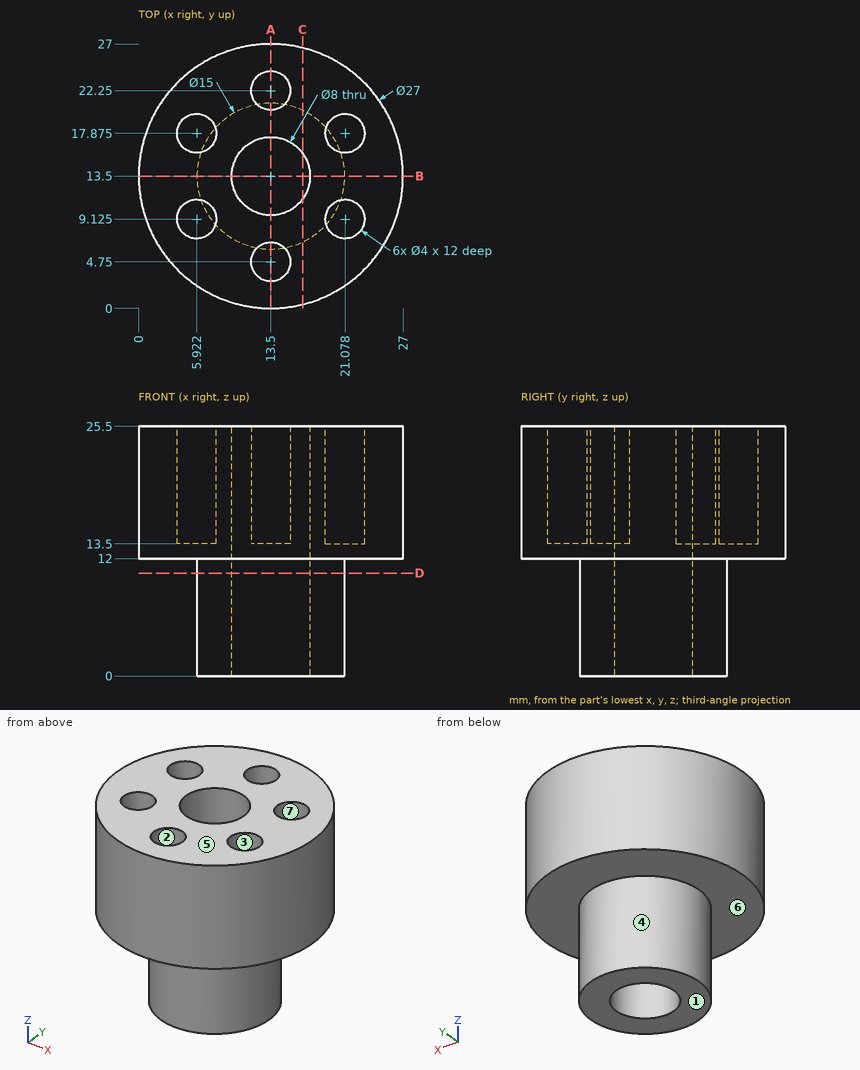
Could you check a few things on this drawing? It's one solid part, dimensions in mm from its lowest x, y, z. A direction names the side the tool comes from. Coordinates: 2 decimals unless noted, no trailing zeros. Order: outer loops, then holes, each group sorted by start corner. A loop starts at its lowest first (then second) coordinate and runs counter-clockwise, first axis right, second up. Notation, with made-up numbers: M 35.5,34 L 40.5,34 A25 ccw 40.5,53 Z; hole C 0.25,57.5 d7. An arc over 180 degrees is marked long. Use a Markdown table: item, result. Add a question column.
Q1. I'm going to push flat-ended pins straight in: pin 1 (2.5 mm diameter, centred on x = 5.92, y = 9.12, fed in from +Z); pin 2 (4 mm diameter, centred on y = 9, z = 20, fed in from -X); pin 3 (1.5 mm diameter, centred on x = 11.5, z = 7.5, fed in from -Y) (1 decimal). Where does each tip first touch, or does it pass through?
Q2. I want a section at B-B on y = 13.5. List the corners of the cut face in (x, z) for me.
Q3. I want a section at C-C on x = 16.75. List the corners of the cut face in (y, z) for me, then the cut area to 3 significant figures.
Q4. I want a section at D-D on z = 10.5. List the corners of the cut face in (x, y) for me, then the cut area to 3 significant figures.
Q5. We'd pull the mould along X, two halves only. Please class the marked faces 1, 2, 3 and 4: pulls with the +X half, pulls with the -X half, needs draft (parallel to the pull), parting line crosses it, or undercut.
Q6. Which directions (+Z, -Z, +X, -X, +Y, -Y) give clear straight access to the entire face, cutting with the end or side of a thin tool? Please do the marked faces 5, 6 and 7.
Q7. If I drill on L1, parallel to X at y = 7.5, z = 24 (1 decimal); L2, parallel to Y at x = 13.5, z = 16; L3, parallel to Y at x = 12.75, z = 20.25 (1 decimal), over which ranges is the centre line in solid material (lowest first)?
Q8. I want a section at A-A on x = 13.5. List the corners of the cut face in (y, z) for me.
Checked values:
| question | item | result |
|---|---|---|
| 1 | pin 1 | z = 13.5 |
| 1 | pin 2 | x = 0.23 |
| 1 | pin 3 | y = 6.1 |
| 2 | outline | M 0,12 L 6,12 L 6,0 L 9.5,0 L 9.5,25.5 L 0,25.5 Z; M 17.5,0 L 21,0 L 21,12 L 27,12 L 27,25.5 L 17.5,25.5 Z |
| 3 | outline | M 0.4,12 L 6.74,12 L 6.74,0 L 11.17,0 L 11.17,25.5 L 0.4,25.5 Z; M 15.83,0 L 20.26,0 L 20.26,12 L 26.6,12 L 26.6,25.5 L 15.83,25.5 Z |
| 3 | area | 397 mm² |
| 4 | outline | C 13.5,13.5 d15; hole C 13.5,13.5 d8 |
| 4 | area | 126 mm² |
| 5 | face 1 | needs draft |
| 5 | face 2 | undercut |
| 5 | face 3 | undercut |
| 5 | face 4 | parting line crosses it |
| 6 | face 5 | +Z, +X, -X, +Y, -Y |
| 6 | face 6 | -Z |
| 6 | face 7 | +Z |
| 7 | L1 | 1.4 to 4.8, 7.1 to 19.9, 22.2 to 25.6 |
| 7 | L2 | 0 to 2.75, 6.75 to 9.5, 17.5 to 20.25, 24.25 to 27 |
| 7 | L3 | 0 to 2.9, 6.6 to 9.6, 17.4 to 20.4, 24.1 to 27 |
| 8 | outline | M 0,12 L 6,12 L 6,0 L 9.5,0 L 9.5,25.5 L 6.75,25.5 L 6.75,13.5 L 2.75,13.5 L 2.75,25.5 L 0,25.5 Z; M 17.5,0 L 21,0 L 21,12 L 27,12 L 27,25.5 L 24.25,25.5 L 24.25,13.5 L 20.25,13.5 L 20.25,25.5 L 17.5,25.5 Z |
